Here's how the part is built. I have some questions about the finished solid (model axes, mm). Face numbers are marked on the shaded views. Coordinates: 2 decimals unless noted, no trailing zeros. Order: outer loops, then holes, each group sorted by start corner. A loop starts at its lowest first (then second) coordinate and runs counter-clockwise, first axis right, second up. Notation, with made-up numbers: M -21,89.25 L -3,89.25 A16 cw -3,119.25 Z; hole C -3.75,-11 d11. An arc over 180 degrees is marked long. Answer as CSV lines item,"result". Start each with the question number.
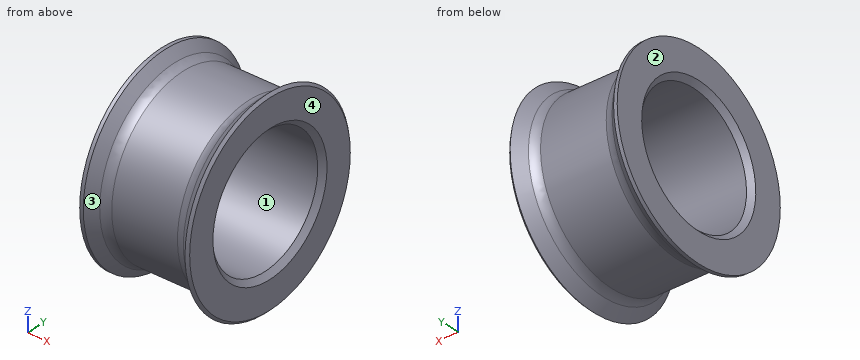
```python
from build123d import *
from OCP.BRepFilletAPI import BRepFilletAPI_MakeChamfer

# Parameters (mm, degrees)
CHAMFER1_SIZE  = 0.2
CHAMFER1_SIZE2 = 0.141421356
FILLET1_R      = 0.5


with BuildPart() as part:
    # Sketch1 → Revolve1 (revolve)
    with BuildSketch(Plane.XY, mode=Mode.PRIVATE) as revolve1_sk:
        Polygon((0, 3.36), (1.5, 3.36), (2.14, 4), (2.14, 2.5), (-2.14, 2.5), (-2.14, 4), (-1.5, 3.36), align=None)
    revolve(revolve1_sk.sketch.rotate(Axis((0, 0, 0), (1, 0, 0)), 90), axis=Axis((0, 0, 0), (1, 0, 0)))

    # Chamfer1: one chamfer whose edges measure the first distance from different faces: ONE call of the kernel's chamfer builder (chamfer() names one face for all edges)
    chamfer1_edges_1 = [part.edges().sort_by_distance(p)[0] for p in [
        (-2.14, 0, -4),
    ]]
    chamfer1_side_1 = [part.faces().sort_by_distance(p)[0] for p in [
        (-1.82, 0, -3.68),
    ]]
    chamfer1_edges_2 = [part.edges().sort_by_distance(p)[0] for p in [
        (-2.14, 0, -2.5),
        (2.14, 0, -2.5),
    ]]
    chamfer1_edges_3 = [part.edges().sort_by_distance(p)[0] for p in [
        (2.14, 0, -4),
    ]]
    chamfer1_side_3 = [part.faces().sort_by_distance(p)[0] for p in [
        (2.14, 0, -3.886862915),
    ]]
    chamfer1 = BRepFilletAPI_MakeChamfer(part.part.solid().wrapped)
    for e in chamfer1_edges_1:
        chamfer1.Add(CHAMFER1_SIZE, CHAMFER1_SIZE2, e.wrapped, chamfer1_side_1[0].wrapped)  # the first distance lies on this face
    for e in chamfer1_edges_2:
        chamfer1.Add(CHAMFER1_SIZE, e.wrapped)
    for e in chamfer1_edges_3:
        chamfer1.Add(CHAMFER1_SIZE, CHAMFER1_SIZE2, e.wrapped, chamfer1_side_3[0].wrapped)  # the first distance lies on this face
    add(Compound.cast(chamfer1.Shape()), mode=Mode.REPLACE)

    # Fillet1
    fillet1_edges = [part.edges().sort_by_distance(p)[0] for p in [
        (-1.5, 0, -3.36),
        (1.5, 0, -3.36),
    ]]
    fillet(fillet1_edges, radius=FILLET1_R)


solid = part.part
```
1) Will these pins go through, and if not, where does the flat tip stop? pin 1 Ø1 at (x, z) = (-0.5, -2.5) entering from +Y; pin 2 Ø1.5 at (x, z) = (0.5, -2.5) entering from +Y.
2) Suppose I cut it at A-A on x = 0. Please give me the cut outline in (y, z), plus the area to 3 significant figures.
3) I need wall thicknesses on line 1 (Y direction, x = 0.3, z = 0); line 2 (Y direction, x = -1.9, z = -1.5); line 3 (X direction, y = -0.75, z = 3.75). Which ranges of each line are inside material? Lowest first, please. Write a range as [from, to].
4) If we mould it in two halves opening along X, with no side actions, what happens to the marked faces 1, 2, 3 and 4? For each: released by +X, released by -X, zero draft, split by the parting line, or undercut.
Output:
1,pin 1,"y = 2.7"
1,pin 2,"y = 2.87"
2,outline,"C 0,0 d6.72; hole C 0,0 d5"
2,area,"15.8 mm²"
3,line 1,"[-3.36, -2.5], [2.5, 3.36]"
3,line 2,"[-3.45, -2], [2, 3.45]"
3,line 3,"[-2.14, -1.96], [1.96, 2.12]"
4,face 1,"zero draft"
4,face 2,"released by -X"
4,face 3,"undercut"
4,face 4,"released by +X"
